Work out the finished part from the listing and answer in its coordinate system (mm). A direction names the side the tool comes from. Round coordinates to 2 decimals unless told otherwise and drop trailing zeros. Order: outer loops, then holes, each group sorted by start corner. A loop starts at its lowest first (then second) coordinate and runs counter-clockwise, first axis right, second up.
from build123d import *

# Parameters (mm, degrees)
SKETCH3_W           = 420
SKETCH3_H           = 760
BOSS_EXTRUDE1_DEPTH = 2
SKETCH7_W           = 380
SKETCH7_H           = 2
BOSS_EXTRUDE2_DEPTH = 420
SKETCH9_W           = 382
SKETCH9_H           = 2
BOSS_EXTRUDE3_DEPTH = 420


with BuildPart() as part:
    # Sketch3 → Boss-Extrude1 (new body)
    with BuildSketch(Plane.XY):
        with Locations((210, 380)):
            Rectangle(SKETCH3_W, SKETCH3_H)
    extrude(amount=BOSS_EXTRUDE1_DEPTH)

    # Sketch7 → Boss-Extrude2 (add)
    with BuildSketch(Plane(origin=(420, 760, 0), x_dir=(0, 0, 1), z_dir=(-1, 0, 0))):
        with Locations((190, 1)):
            Rectangle(SKETCH7_W, SKETCH7_H)
    extrude(amount=BOSS_EXTRUDE2_DEPTH)

    # Sketch9 → Boss-Extrude3 (add)
    with BuildSketch(Plane(origin=(420, 0, 2), x_dir=(0, 0, -1), z_dir=(1, 0, 0))):
        with Locations((-189, 1)):
            Rectangle(SKETCH9_W, SKETCH9_H)
    extrude(amount=-BOSS_EXTRUDE3_DEPTH)


solid = part.part
Item 1: Given pin 1 (1 mm diameter, centred on x = 132, y = 761.5, fed in from +Z); pin 2 (1 mm diameter, centred on x = 69.5, y = 253, fed in from +Z), each flat-ended and moving along its own axis, determine where each tip first touches the part or whether it passes through.
Item 2: Find section C-C (y = 194). Write down the section's boundary in (x, z), plus the area to 3 significant figures.
Item 3: Find section A-A (x = 362). Write down the section's boundary in (y, z).
Item 4: For a pull along Y with two mould halves and no side action, classify faces 3 (the face through (213, 762, 187)), 4 (the face through (213, 376, 0)), 5 (the face through (207, 386, 2)) as released by +Y, released by -Y, zero draft, split by the parting line, or undercut.
Item 5: Find section B-B (z = 39). Write down the section's boundary in (x, y), plus the area to 3 significant figures.
Item 6: A tool of negligible diameter and unlimited length cuts with its end or side. For faces 1 (the face through (213, 2, 195)), 2 (the face through (213, 0, 194)), from which of +Z, -Z, +X, -X, +Y, -Y can it reach the whole face along a straight path? Write none if from no direction.
Item 7: Find the intervals of material crossed by line 1 along Y through (x, z) = (395.5, 324); line 2 along Z through (x, y) = (68, 662), in increasing order.
Model answer:
1. pin 1: stops at z = 380
1. pin 2: stops at z = 2
2. outline: (0, 0) - (420, 0) - (420, 2) - (0, 2) - close
2. area: 840 mm2
3. outline: (0, 0) - (762, 0) - (762, 380) - (760, 380) - (760, 2) - (2, 2) - (2, 382) - (0, 382) - close
4. face 3: released by +Y
4. face 4: zero draft
4. face 5: undercut
5. outline: (0, 0) - (420, 0) - (420, 2) - (0, 2) - close; (0, 760) - (420, 760) - (420, 762) - (0, 762) - close
5. area: 1,680 mm2
6. face 1: +Z, +X, -X
6. face 2: +Z, -Z, +X, -X, -Y
7. line 1: y = 0 to 2, 760 to 762
7. line 2: z = 0 to 2
